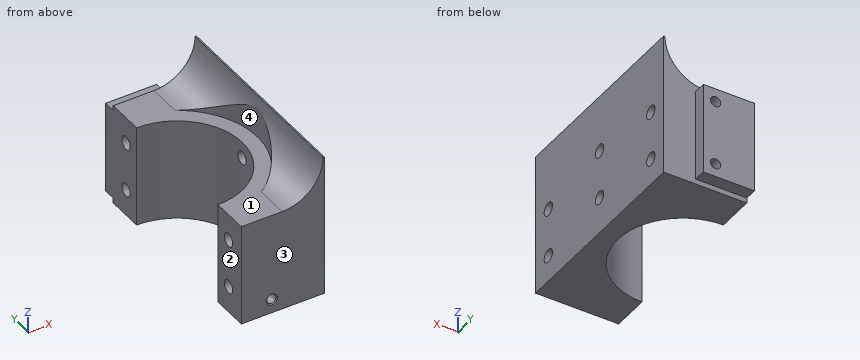
```python
from build123d import *

# Parameters (mm, degrees)
CENTRE_HOLE_FOR_L2_DEPTH      = 40
CENTRE_HOLE_FOR_L2_DEPTH_BACK = 10
SKETCH1_R                     = 39.1
SKETCH1_R_2                   = 31.75
MAIN_STRUCTURE_DEPTH          = 60
MAIN_STRUCTURE_DEPTH_BACK     = 50
SKETCH2_W                     = 100
SKETCH2_H                     = 100
SKETCH2_R                     = 39.1
BEARING_CURVE_DEPTH           = 10
SKETCH6_R                     = 10.5
SHAFT_HOLE_DEPTH              = 10
WRIST_CUTOUT_DEPTH            = 188.082869339
SKETCH11_W                    = 25
SKETCH11_H                    = 45
SKETCH11_R                    = 2.525
BOSS_EXTRUDE1_DEPTH           = 6
CUT_EXTRUDE6_DEPTH            = 168.73789077
CUT_EXTRUDE6_DEPTH_BACK       = 168.73789077
SKETCH18_R                    = 3.25
CUT_EXTRUDE7_START            = -1.5875
CUT_EXTRUDE7_DEPTH            = 1.5875
SKETCH9_R                     = 12.05
BEARING_DEPTH                 = 5
CUT_EXTRUDE8_DEPTH            = 3
SKETCH21_R                    = 3.25
SKETCH21_R_2                  = 1.65
CUT_EXTRUDE9_DEPTH            = 167.868211501
CUT_EXTRUDE10_DEPTH           = 6.35
SKETCH23_R                    = 2.275
CUT_EXTRUDE11_DEPTH           = 6
CHAMFER1_SIZE                 = 0.5


with BuildPart() as part:
    # Sketch1 → Centre Hole for L2 (new, two sides: drawn at the far end of the back side and taken through both)
    with BuildSketch(Plane.XY.offset(-CENTRE_HOLE_FOR_L2_DEPTH_BACK)):
        Circle(SKETCH1_R)
        Circle(SKETCH1_R_2, mode=Mode.SUBTRACT)
    extrude(amount=CENTRE_HOLE_FOR_L2_DEPTH + CENTRE_HOLE_FOR_L2_DEPTH_BACK)

    # Sketch2 → Main Structure (add, two sides: drawn at the far end of the back side and taken through both)
    with BuildSketch(Plane.XY.offset(40).offset(-MAIN_STRUCTURE_DEPTH_BACK)):
        Rectangle(SKETCH2_W, SKETCH2_H)
        Circle(SKETCH2_R, mode=Mode.SUBTRACT)
    extrude(amount=MAIN_STRUCTURE_DEPTH + MAIN_STRUCTURE_DEPTH_BACK)

    # Sketch3 → Bearing Curve (add)
    with BuildSketch(Plane.ZY.offset(50)):
        with BuildLine():
            Line((100, 50), (100, -50))
            ThreePointArc((100, -50), (150, 0), (100, 50))
        make_face()
    bearing_curve = extrude(amount=-BEARING_CURVE_DEPTH)

    # Upright Mirror: Bearing Curve across plane
    add(bearing_curve.mirror(Plane(origin=(0, 0, 0), x_dir=(0, 0, 1), z_dir=(1, 0, 0))))

    # Sketch6 → Shaft Hole (cut)
    with BuildSketch(Plane.ZY.offset(50)):
        with Locations((100, 0)):
            Circle(SKETCH6_R)
    extrude(amount=-SHAFT_HOLE_DEPTH, mode=Mode.SUBTRACT)

    # Sketch4 → Wrist Cutout (cut, through all)
    with BuildSketch(Plane(origin=(0, 50, 0), x_dir=(1, 0, 0), z_dir=(0, 1, 0))):
        with BuildLine():
            Line((-40, -100), (-40, -60))
            ThreePointArc((-40, -60), (-34.142135624, -45.857864376), (-20, -40))
            Line((-20, -40), (20, -40))
            ThreePointArc((20, -40), (34.142135624, -45.857864376), (40, -60))
            Line((40, -60), (40, -100))
            Line((40, -100), (-40, -100))
        make_face()
    extrude(amount=-WRIST_CUTOUT_DEPTH, mode=Mode.SUBTRACT)

    # SurfaceCut1
    split(bisect_by=Plane.ZY, keep=Keep.TOP)

    # Sketch11 → Boss-Extrude1 (add)
    with BuildSketch(Plane(origin=(0, 50, 0), x_dir=(1, 0, 0), z_dir=(0, 1, 0))):
        with Locations((-12.5, -15)):
            Rectangle(SKETCH11_W, SKETCH11_H)
        with Locations(Location((-19, 1, 0), (0, 0, 270))):
            Circle(SKETCH11_R, mode=Mode.SUBTRACT)
        with Locations(Location((-19, -31, 0), (0, 0, 270))):
            Circle(SKETCH11_R, mode=Mode.SUBTRACT)
    extrude(amount=BOSS_EXTRUDE1_DEPTH)

    # Sketch18 → Cut-Extrude6 (cut, two sides: drawn at the far end of the back side and taken through both)
    with BuildSketch(Plane.ZY.offset(50).offset(-CUT_EXTRUDE6_DEPTH_BACK)):
        with Locations((8, 0)):
            Circle(SKETCH18_R)
        with Locations((32, 0)):
            Circle(SKETCH18_R)
    extrude(amount=CUT_EXTRUDE6_DEPTH + CUT_EXTRUDE6_DEPTH_BACK, mode=Mode.SUBTRACT)

    # Sketch19 → Cut-Extrude7 (cut)
    with BuildSketch(Plane(origin=(-40, 0, 0), x_dir=(0, 0, -1), z_dir=(1, 0, 0)).offset(CUT_EXTRUDE7_START)):
        with BuildLine():
            Line((-60, 50), (-100, 50))
            ThreePointArc((-100, 50), (-150, 0), (-100, -50))
            Line((-100, -50), (-60, -50))
            Line((-60, -50), (-60, 50))
        make_face()
    extrude(amount=CUT_EXTRUDE7_DEPTH, mode=Mode.SUBTRACT)

    # Sketch9 → Bearing (cut)
    with BuildSketch(Plane(origin=(-41.5875, 0, 0), x_dir=(0, 0, -1), z_dir=(1, 0, 0))):
        with Locations((-100, 0)):
            Circle(SKETCH9_R)
    extrude(amount=-BEARING_DEPTH, mode=Mode.SUBTRACT)

    # Sketch20 → Cut-Extrude8 (cut)
    with BuildSketch(Plane.ZY.offset(50)):
        with BuildLine():
            Line((-10, -50), (100, -50))
            ThreePointArc((100, -50), (150, 0), (100, 50))
            Line((100, 50), (-10, 50))
            Line((-10, 50), (-10, -50))
        make_face()
    extrude(amount=-CUT_EXTRUDE8_DEPTH, mode=Mode.SUBTRACT)

    # Sketch21 → Cut-Extrude9 (cut, through all)
    with BuildSketch(Plane.ZY.offset(47)):
        with Locations((3, -40)):
            Circle(SKETCH21_R)
        with Locations((27, -40)):
            Circle(SKETCH21_R)
        with Locations(Location((27, 40, 0), (0, 0, 180))):
            Circle(SKETCH21_R)
        with Locations(Location((3, 40, 0), (0, 0, 180))):
            Circle(SKETCH21_R)
        with Locations((125, 0)):
            Circle(SKETCH21_R_2)
    extrude(amount=-CUT_EXTRUDE9_DEPTH, mode=Mode.SUBTRACT)

    # Sketch22 → Cut-Extrude10 (cut)
    with BuildSketch(Plane.ZY.offset(47)):
        with BuildLine():
            Line((-10, 50), (-10, -50))
            Line((-10, -50), (100, -50))
            ThreePointArc((100, -50), (150, 0), (100, 50))
            Line((100, 50), (-10, 50))
        make_face()
    extrude(amount=-CUT_EXTRUDE10_DEPTH, mode=Mode.SUBTRACT)

    # Sketch23 → Cut-Extrude11 (cut)
    with BuildSketch(Plane(origin=(0, -50, 0), x_dir=(-1, 0, 0), z_dir=(0, -1, 0))):
        with Locations(Location((15, 3.25, 0), (0, 0, 90))):
            Circle(SKETCH23_R)
    extrude(amount=-CUT_EXTRUDE11_DEPTH, mode=Mode.SUBTRACT)

    # Chamfer1
    chamfer1_edges = [part.edges().sort_by_distance(p)[0] for p in [
        (-15, -50, -0.975),
    ]]
    chamfer(chamfer1_edges, length=CHAMFER1_SIZE)


with BuildPart() as body_2:
    # Mirror1: mirrored copy
    add(part.part.mirror(Plane.ZY))


solid = body_2.part
```
Work out the finished part from the listing and answer in its coordinate system (mm). Face numbers are marked on the shaded views. Round coordinates to 2 decimals unless told otherwise and drop trailing zeros. Loops run counter-clockwise (first coordinate to the right, second up) from the corner with the lowest first, then second, coordinate; pieces in that order, holes last.
(1) The mould has two halves that part along Y. Classify the marked faces 1, 2, 3 and 4: pulls with the +Y half, pulls with the -Y half, needs draft (parallel to the pull), parting line crosses it, or undercut.
Computed values:
face 1: undercut
face 2: needs draft
face 3: pulls with the -Y half
face 4: undercut
(2) The part is cut by section B-B, the plane z = 3. Give the vertices of the cut face in (x, y), and give its area (3 significant figures).
Computed values:
outline: (0, -50) - (40.65, -50) - (40.65, -43.25) - (0, -43.25) - close; (0, -36.75) - (40.65, -36.75) - (40.65, 36.75) - (0, 36.75) - (0, 31.75) arc R31.75 cw to (0, -31.75) - close; (0, 43.25) - (40.65, 43.25) - (40.65, 50) - (25, 50) - (25, 56) - (0, 56) - close
area: 2,100 mm2
(3) The part is cut by section A-A, the plane y = -40. Give the vertices of the cut face in (x, z).
Computed values:
outline: (0, -10) - (40.65, -10) - (40.65, -0.25) - (0, -0.25) - close; (0, 6.25) - (40.65, 6.25) - (40.65, 23.75) - (0, 23.75) - close; (0, 30.25) - (40.65, 30.25) - (40.65, 60) - (40, 60) arc R20 cw to (20, 40) - (0, 40) - close
(4) The part is cut by section C-C, the plane x = 23. Give the vertices of the cut face in (y, z).
Computed values:
outline: (-50, -10) - (-21.89, -10) - (-21.89, 40) - (-31.62, 40) - (-31.62, 40.23) - (-50, 40.23) - close; (21.89, -10) - (50, -10) - (50, -7.5) - (56, -7.5) - (56, 37.5) - (50, 37.5) - (50, 40.23) - (31.62, 40.23) - (31.62, 40) - (21.89, 40) - close; hole circle Ø6.5 at (-40, 3); hole circle Ø6.5 at (-40, 27); hole circle Ø6.5 at (40, 3); hole circle Ø6.5 at (40, 27)
(5) Find the intervals of material crossed by L1, parallel to Z at x = 35, y = 0; L2, parallel to Z at x = 6.5, y = -40.5; L3, parallel to Y at x = 38, z = 24, in increasing order.
Computed values:
L1: z = -10 to 4.75, 11.25 to 28.75, 35.25 to 40
L2: z = -10 to -0.21, 6.21 to 23.79, 30.21 to 40
L3: y = -50 to -41.25, -38.75 to 38.75, 41.25 to 50
(6) Each of these flat-tipped pins is pushed along its axis until it touches: P1, Ø4, axis at x = 19, z = 31, coming from the +Y side; P2, Ø1.8, axis at x = 6.5, y = 53.5, coming from the +Z side; P3, Ø6, axis at x = 16, y = 33, coming from the +Z side. Where does it stop, or does it pass through?
Computed values:
P1: stops at y = 50
P2: stops at z = 37.5
P3: stops at z = 40
(7) The part is cut by section D-D, the plane y = 0. Give the vertices of the cut face in (x, z), and give its area (3 significant figures).
Computed values:
outline: (31.75, -10) - (40.65, -10) - (40.65, 4.75) - (31.75, 4.75) - close; (31.75, 11.25) - (40.65, 11.25) - (40.65, 28.75) - (31.75, 28.75) - close; (31.75, 35.25) - (40.65, 35.25) - (40.65, 60) - (40, 60) arc R20 cw to (39.1, 54.07) - (39.1, 40) - (31.75, 40) - close
area: 357 mm2
